Geometry check sheet. Reference: the model listing, model coordinates, mm. Round coordinates to 2 decimals unless told otherwise and drop trailing zeros. Write each loop counter-clockwise with the first axis right and the second up, starting at its lowest first coordinate (ties: lowest second). Pieces come first, ordered by that corner, then holes.
Item 1: Cross-section at B-B (z = 4). Enter the section's corners in (x, y).
Item 2: Scan lines: probe 1 along X at (y, z) = (-26, 7); probe 2 along X at (y, z) = (-23.5, 4.25); probe 3 along X at (y, z) = (19.5, 1). Record each from-to range of solid material in increasing order.
Item 3: Cross-section at D-D (y = 39.5). Enter the section's corners in (x, z).
Item 4: Cross-section at C-C (y = -26.5). Enter the section's corners in (x, z), then the cut area to 3 significant figures.
Item 5: Cross-section at A-A (x = -44). Enter the section's corners in (y, z).
Item 6: Depth check by flat-ended pin: P1, Ø1.6, axis at x = 43.5, z = 4.5, coming from the +Y side; P2, Ø5, axis at y = -29, z = 8.5, coming from the +X side. Enter the tip coordinate at first touch or a pass-through.
from build123d import *

# Parameters (mm, degrees)
F0_W     = 120
F0_H     = 100
F1_DEPTH = 10
F2_W     = 10
F2_H     = 30
F3_DEPTH = 10.001
F5_DEPTH = 25


with BuildPart() as f1:
    # F0 (on Top) → F1 (new body)
    with BuildSketch(Plane.XY):
        Rectangle(F0_W, F0_H)
    extrude(amount=F1_DEPTH)

    # F2 (on face) → F3 (cut, through all)
    with BuildSketch(Plane.XY.offset(10)):
        with Locations((-45, -25)):
            Rectangle(F2_W, F2_H)
    extrude(amount=-F3_DEPTH, mode=Mode.SUBTRACT)

    # F4 (on face) → F5 (cut)
    with BuildSketch(Plane.XY.offset(10)):
        Polygon((45, -50), (60, -50), (60, 50), (41.829597, 50), (41.829597, 37.5), (45, 37.5), (45, 25), (41.829597, 25), (41.829597, 12.5), (45, 12.5), (45, 0), (41.829597, 0), (41.829597, -12.5), (45, -12.5), (45, -25), (41.829597, -25), (41.829597, -37.5), (45, -37.5), align=None)
    extrude(amount=-F5_DEPTH, mode=Mode.SUBTRACT)


solid = f1.part
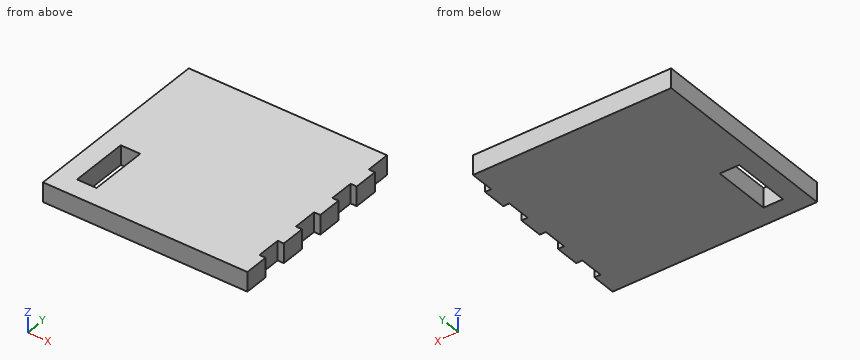
Resolved:
1. outline: (-60, -50) - (45, -50) - (45, -37.5) - (41.83, -37.5) - (41.83, -25) - (45, -25) - (45, -12.5) - (41.83, -12.5) - (41.83, 0) - (45, 0) - (45, 12.5) - (41.83, 12.5) - (41.83, 25) - (45, 25) - (45, 37.5) - (41.83, 37.5) - (41.83, 50) - (-60, 50) - close; hole (-50, -40) - (-40, -40) - (-40, -10) - (-50, -10) - close
2. probe 1: x = -60 to -50, -40 to 41.83
2. probe 2: x = -60 to -50, -40 to 45
2. probe 3: x = -60 to 41.83
3. outline: (-60, 0) - (41.83, 0) - (41.83, 10) - (-60, 10) - close
4. outline: (-60, 0) - (-50, 0) - (-50, 10) - (-60, 10) - close; (-40, 0) - (41.83, 0) - (41.83, 10) - (-40, 10) - close
4. area: 918 mm2
5. outline: (-50, 0) - (-40, 0) - (-40, 10) - (-50, 10) - close; (-10, 0) - (50, 0) - (50, 10) - (-10, 10) - close
6. P1: stops at y = 37.5
6. P2: stops at x = 41.83
